Could you check a few things on this model? Use its own coordinates, in mm. Face numbers are marked on the shaded views. Give positions to 0.01 mm unless a question says otherwise; leave off trailing zeros. Order: outer loops, then holes, each group sorted by start corner. A loop starts at its lowest first (then second) coordinate and runs counter-clockwise, first axis right, second up.
(1) If I drill on probe 1 along X at (y, z) = (1.5, 1.15); probe 2 along X at (y, z) = (2.5, 3.2); probe 3 along Y at (x, z) = (49.2, 3.3), over which ranges is the centre line in solid material (lowest first)?
(2) Imagine slicing it at D-D, the plane y = 5. Write out the boundary of the cut face in (x, z), then the cut area to 3 significant figures.
(3) If we mould it in two halves opening along Y, with no side actions, what happens to the marked faces 1, 2, 3 and 4? For each: released by +Y, released by -Y, zero draft, split by the parting line, or undercut.
(4) Imagine slicing it at C-C, the plane y = -3.25. Write out the boundary of the cut face in (x, z), then the cut area to 3 significant figures.
(5) Imagine slicing it at A-A, the plane y = 0. Write out the boundary of the cut face in (x, z), then the cut area to 3 significant figures.
(6) Will these pins go through, and if not, where does the flat tip stop? pin 1 (6 mm diameter, centred on x = 24.5, y = -2.5, fed in from -Z); pin 2 (2 mm diameter, centred on y = 3, z = 1.5, fed in from +X).
(7) Imagine slicing it at B-B, the plane z = 3.6. Write out the boundary of the cut face in (x, y).
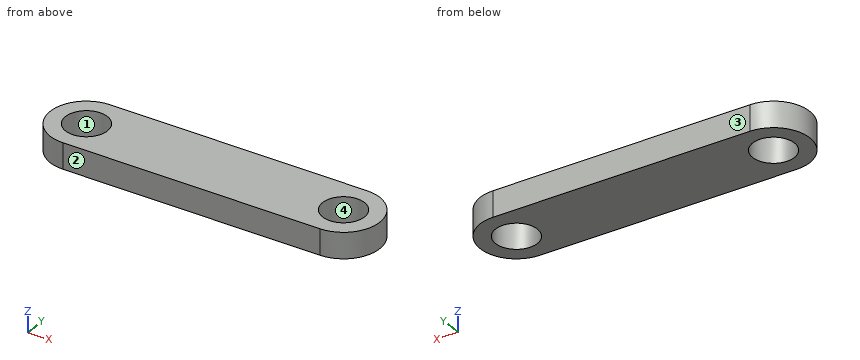
from build123d import *

# Parameters (mm, degrees)
SKETCH_1_R      = 7
SKETCH_1_R_2    = 4.05
EXTRUDE_1_DEPTH = 5


with BuildPart() as part:
    # 草图1 → 凸台-拉伸1 (new body)
    # profile 1 of 3: a face of its own
    with BuildSketch(Plane.XY):
        with BuildLine():
            ThreePointArc((7, 0), (4.949747468, -4.949747468), (0, -7))
            Line((0, -7), (49.2, -7))
            ThreePointArc((49.2, -7), (42.2, 0), (49.2, 7))
            Line((49.2, 7), (0, 7))
            ThreePointArc((0, 7), (4.949747468, 4.949747468), (7, 0))
        make_face()
    # profile 2 of 3: a face of its own
    with BuildSketch(Plane.XY):
        Circle(SKETCH_1_R)
        Circle(SKETCH_1_R_2, mode=Mode.SUBTRACT)
    # profile 3 of 3: a face of its own
    with BuildSketch(Plane.XY):
        with Locations((49.2, 0)):
            Circle(SKETCH_1_R)
        with Locations((49.2, 0)):
            Circle(SKETCH_1_R_2, mode=Mode.SUBTRACT)
    extrude(amount=EXTRUDE_1_DEPTH)


solid = part.part
Answer block:
1. probe 1: x = -6.84 to -3.76, 3.76 to 45.44, 52.96 to 56.04
1. probe 2: x = -6.54 to -3.19, 3.19 to 46.01, 52.39 to 55.74
1. probe 3: y = -7 to -4.05, 4.05 to 7
2. outline: (-4.9, 0) - (54.1, 0) - (54.1, 5) - (-4.9, 5) - close
2. area: 295 mm2
3. face 1: undercut
3. face 2: released by -Y
3. face 3: released by +Y
3. face 4: undercut
4. outline: (-6.2, 0) - (-2.42, 0) - (-2.42, 5) - (-6.2, 5) - close; (2.42, 0) - (46.78, 0) - (46.78, 5) - (2.42, 5) - close; (51.62, 0) - (55.4, 0) - (55.4, 5) - (51.62, 5) - close
4. area: 260 mm2
5. outline: (-7, 0) - (-4.05, 0) - (-4.05, 5) - (-7, 5) - close; (4.05, 0) - (45.15, 0) - (45.15, 5) - (4.05, 5) - close; (53.25, 0) - (56.2, 0) - (56.2, 5) - (53.25, 5) - close
5. area: 235 mm2
6. pin 1: stops at z = 0
6. pin 2: stops at x = 55.91
7. outline: (0, -7) - (49.2, -7) arc R7 ccw to (49.2, 7) - (0, 7) arc R7 ccw to start; hole circle Ø8.1 at (0, 0); hole circle Ø8.1 at (49.2, 0)
